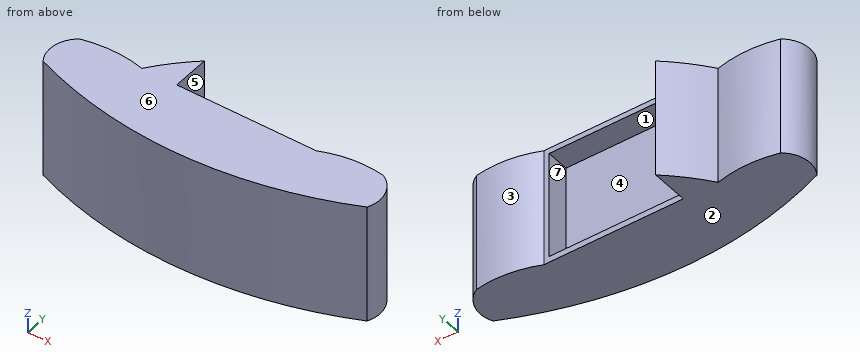
from build123d import *

# Parameters (mm, degrees)
BOSS_EXTRUDE2_DEPTH     = 121.666
SKETCH4_W               = 132.653422834
SKETCH4_H               = 110.004689212
CUT_EXTRUDE1_DEPTH      = 34.29
CUT_EXTRUDE1_DEPTH_BACK = 23.368


with BuildPart() as part:
    # Sketch2 → Boss-Extrude2 (new body)
    with BuildSketch(Plane.XY):
        with BuildLine():
            Line((88.9, 0), (-53.34, 0))
            Line((-53.34, 0), (-53.34, 38.074701195))
            ThreePointArc((-53.34, 38.074701195), (-72.236919303, 20.080501277), (-88.9, 0))
            ThreePointArc((-88.9, 0), (-120.65, 4.094872711), (-152.4, 0))
            ThreePointArc((-152.4, 0), (-164.191323146, -18.853572603), (-159.736653386, -40.64))
            ThreePointArc((-159.736653386, -40.64), (3.572889221, -70.366104417), (165.383346614, -33.33876494))
            ThreePointArc((165.383346614, -33.33876494), (166.92020334, -10.301221175), (151.978855147, 7.30123506))
            ThreePointArc((151.978855147, 7.30123506), (119.904882148, 8.268810644), (88.9, 0))
        make_face()
    extrude(amount=BOSS_EXTRUDE2_DEPTH)

    # Sketch4 → Cut-Extrude1 (cut, two sides)
    with BuildSketch(Plane(origin=(0, 0, 0), x_dir=(1, 0, 0), z_dir=(0, 1, 0))) as cut_extrude1_sk:
        with Locations((17.235431011, -61.044907142)):
            Rectangle(SKETCH4_W, SKETCH4_H)
    extrude(amount=CUT_EXTRUDE1_DEPTH, mode=Mode.SUBTRACT)
    extrude(cut_extrude1_sk.sketch, amount=-CUT_EXTRUDE1_DEPTH_BACK, mode=Mode.SUBTRACT)


solid = part.part
The listing builds one solid part. Answer for the finished solid, in the listing's coordinates (mm). Face numbers are marked on the shaded views. A direction names the side the tool comes from. Round coordinates to 2 decimals unless told otherwise and drop trailing zeros. Order: outer loops, then holes, each group sorted by start corner. A loop starts at its lowest first (then second) coordinate and runs counter-clockwise, first axis right, second up. Notation, with made-up numbers: (-16, 83.5) -> (30, 83.5) arc R15 ccw to (30, 87.5) -> close; hole circle Ø4 at (22.25, -23.5). An arc over 180 degrees is marked (long way). One line per item, written item: value.
Item 1: Find section B-B, the plane z = 13. Give the vertices of the cut face in (x, y).
Taken from the geometry:
outline: (-159.74, -40.64) arc R412.66 ccw to (165.38, -33.34) arc R30.72 ccw to (151.98, 7.3) arc R110.74 ccw to (88.9, 0) -> (83.56, 0) -> (83.56, -23.37) -> (-49.09, -23.37) -> (-49.09, 0) -> (-53.34, 0) -> (-53.34, 38.07) arc R222.76 ccw to (-88.9, 0) arc R125.14 ccw to (-152.4, 0) arc R29.95 ccw to start
Item 2: Given P1, Ø6, axis at x = -10.5, z = 70, coming from the +Y side; P2, Ø11.5, axis at y = -13.5, z = 58, coming from the -X side; P3, Ø10, axis at x = 70, z = 87, coming from the -Y side, each flat-ended and moving along its own axis, determine where each tip first touches the part or whether it passes through.
Taken from the geometry:
P1: stops at y = -23.37
P2: stops at x = -164.26
P3: stops at y = -64.37
Item 3: For a pull along Z with two mould halves and no side action, classify the marked faces 1, 2, 3 and 4 as released by +Z, released by -Z, zero draft, split by the parting line, or undercut.
Taken from the geometry:
face 1: undercut
face 2: released by -Z
face 3: zero draft
face 4: undercut
Item 4: Find section D-D, the plane x = 35. Give the vertices of the cut face in (y, z), then the cut area to 3 significant figures.
Taken from the geometry:
outline: (-68.46, 0) -> (0, 0) -> (0, 6.04) -> (-23.37, 6.04) -> (-23.37, 116.05) -> (0, 116.05) -> (0, 121.67) -> (-68.46, 121.67) -> close
area: 5,760 mm2
Item 5: Find section C-C, the plane x = -28. Give the vertices of the cut face in (y, z).
Taken from the geometry:
outline: (-69.87, 0) -> (0, 0) -> (0, 6.04) -> (-23.37, 6.04) -> (-23.37, 116.05) -> (0, 116.05) -> (0, 121.67) -> (-69.87, 121.67) -> close
Item 6: Straight lines are drawn through the part: L1, parallel to X at y = -2.5, z = 9; L2, parallel to Y at x = 1, z = 85.5; L3, parallel to X at y = -11, z = 82. For each, find the intervals that lie inside material, in ascending order.
Taken from the geometry:
L1: x = -155.39 to -49.09, 83.56 to 163.05
L2: y = -70.42 to -23.37
L3: x = -161.61 to -49.09, 83.56 to 167.14
Item 7: For the marked faces 5, 6 and 7, determine the directions among +Z, -Z, +X, -X, +Y, -Y from which every point of the face is accessible in a straight line to the end or side of a thin tool.
Taken from the geometry:
face 5: +Z, -Z, +Y
face 6: +Z, +X, -X, +Y, -Y
face 7: +Y
Item 8: Find section A-A, the plane y = -3.5. Give the vertices of the cut face in (x, z).
Taken from the geometry:
outline: (-156.39, 0) -> (163.71, 0) -> (163.71, 121.67) -> (-156.39, 121.67) -> close; hole (-49.09, 6.04) -> (83.56, 6.04) -> (83.56, 116.05) -> (-49.09, 116.05) -> close
